```python
from build123d import *

# Parameters (mm, degrees)
SKETCH1_W           = 23.056445047489827
SKETCH1_H           = 95.25
SKETCH1_R           = 1.2700000000000005
SKETCH1_R_2         = 1.269999999999998
BOSS_EXTRUDE1_DEPTH = 6.35
SKETCH2_W           = 23.056445047489827
SKETCH2_H           = 48.26
BOSS_EXTRUDE2_DEPTH = 12.7
CUT_EXTRUDE2_DEPTH  = 55.41534970233967
SKETCH6_R           = 3.4289999999999994
CUT_EXTRUDE3_DEPTH  = 53.57321599024526
FILLET2_R           = 1.27
BOSS_EXTRUDE3_DEPTH = 6.35
SKETCH9_R           = 1.9049999999999996
SKETCH9_R_2         = 1.905
CUT_EXTRUDE4_DEPTH  = 53.43149307056342
FILLET4_R           = 2.54
BOSS_EXTRUDE7_DEPTH = 6.35
FILLET5_R           = 2.54
FILLET6_R           = 2.54
SKETCH13_R          = 2.0319999999999987
SKETCH13_R_2        = 2.032000000000001
CUT_EXTRUDE5_DEPTH  = 6.35
FILLET7_R           = 2.54


with BuildPart() as part:
    # Sketch1 → Boss-Extrude1 (new body)
    # profile 1 of 4: a face of its own
    with BuildSketch(Plane.XY):
        Rectangle(SKETCH1_W, SKETCH1_H)
        Polygon((7.9121000000000015, 16.687800000000006), (7.9121000000000015, 44.449999999999996), (-7.912099999999998, 44.45), (-7.912099999999998, 16.687800000000006), align=None, mode=Mode.SUBTRACT)
    # profile 2 of 4: a face of its own
    with BuildSketch(Plane.XY):
        Polygon((-7.912099999999998, 16.687800000000006), (7.9121000000000015, 16.687800000000006), (7.9121000000000015, 44.449999999999996), (-7.912099999999998, 44.45), align=None)
        with Locations((5.372100000000001, 19.227800000000006)):
            Circle(SKETCH1_R, mode=Mode.SUBTRACT)
        with Locations((-5.372099999999998, 41.910000000000004)):
            Circle(SKETCH1_R_2, mode=Mode.SUBTRACT)
    # profile 3 of 4: a face of its own
    with BuildSketch(Plane.XY):
        with Locations((-5.372099999999998, 41.910000000000004)):
            Circle(SKETCH1_R_2)
    # profile 4 of 4: a face of its own
    with BuildSketch(Plane.XY):
        with Locations((5.372100000000001, 19.227800000000006)):
            Circle(SKETCH1_R)
    extrude(amount=BOSS_EXTRUDE1_DEPTH)

    # Sketch2 → Boss-Extrude2 (add)
    with BuildSketch(Plane(origin=(0, 0, 0), x_dir=(-1, 0, 0), z_dir=(0, 0, -1))):
        with Locations((0, -23.495)):
            Rectangle(SKETCH2_W, SKETCH2_H)
    extrude(amount=BOSS_EXTRUDE2_DEPTH)

    # Sketch5 → Cut-Extrude2 (cut, through all)
    with BuildSketch(Plane(origin=(11.528222523744914, 0, 0), x_dir=(0, 0, -1), z_dir=(1, 0, 0))):
        Polygon((-0.6350000000000019, -12.065000000000001), (9.524999999999997, -12.065000000000001), (9.524999999999999, -8.255000000000003), (-0.6350000000000019, -8.255000000000003), align=None)
    extrude(amount=-CUT_EXTRUDE2_DEPTH, mode=Mode.SUBTRACT)

    # Sketch6 → Cut-Extrude3 (cut, through all)
    with BuildSketch(Plane(origin=(0, 0, -12.7), x_dir=(-1, 0, 0), z_dir=(0, 0, -1))):
        with Locations((0, -28.575)):
            Circle(SKETCH6_R)
    extrude(amount=-CUT_EXTRUDE3_DEPTH, mode=Mode.SUBTRACT)

    # Fillet2
    fillet2_edges = [part.edges().sort_by_distance(p)[0] for p in [
        (-11.528222523744914, -10.160000000000004, -9.524999999999999),
        (0, -8.255000000000003, -9.524999999999999),
        (-11.528222523744914, -12.065, -4.444999999999998),
        (0, -12.065000000000001, -9.524999999999997),
        (-11.528222523744914, -10.16, 0.6350000000000019),
        (0, -12.065000000000001, 0.6350000000000019),
        (-11.528222523744914, -8.255000000000003, -4.4449999999999985),
        (0, -8.255000000000003, 0.6350000000000019),
        (11.528222523744914, -10.160000000000002, -9.524999999999999),
        (11.528222523744914, -8.255000000000003, -4.4449999999999985),
        (11.528222523744914, -10.160000000000002, 0.6350000000000019),
        (11.528222523744914, -12.065000000000001, -4.444999999999998),
    ]]
    fillet(fillet2_edges, radius=FILLET2_R)

    # Sketch8 → Boss-Extrude3 (add)
    with BuildSketch(Plane.ZY.offset(11.528222523744914)):
        Polygon((6.35, 47.625), (-1.21e-15, 47.625), (0, 6.98625472546675), (6.350000000000005, 6.986254725466751), align=None)
    extrude(amount=BOSS_EXTRUDE3_DEPTH)

    # Sketch9 → Cut-Extrude4 (cut, through all)
    with BuildSketch(Plane.XY):
        with Locations((-4.594022523744915, 12.877800000000006)):
            Circle(SKETCH9_R)
        with Locations((-15.338222523744914, 35.56)):
            Circle(SKETCH9_R_2)
    extrude(amount=CUT_EXTRUDE4_DEPTH, mode=Mode.SUBTRACT)

    # Fillet4
    fillet4_edges = [part.edges().sort_by_distance(p)[0] for p in [
        (11.528222523744914, 47.625, 3.175),
        (-11.528222523744914, 6.98625472546675, 3.1750000000000025),
        (-17.878222523744913, 47.625, 3.1749999999999994),
        (-17.878222523744913, 6.98625472546675, 3.1750000000000025),
    ]]
    fillet(fillet4_edges, radius=FILLET4_R)

    # Sketch12 → Boss-Extrude7 (add)
    with BuildSketch(Plane(origin=(11.528222523744914, 0, 0), x_dir=(0, 0, -1), z_dir=(1, 0, 0))):
        Polygon((-6.35, 0.6349999999999898), (18.613653389650153, 0.6349999999999898), (18.613653389650153, 9.627193152709879), (-17.78195834691587, 9.627193152709879), (-17.78195834691587, 0.6349999999999898), align=None)
    extrude(amount=-BOSS_EXTRUDE7_DEPTH)

    # Fillet5
    fillet5_edges = [part.edges().sort_by_distance(p)[0] for p in [
        (8.353222523744913, 0.6349999999999967, -12.7),
        (8.353222523744915, 9.627193152709879, 6.3500000000000005),
        (8.353222523744915, 9.627193152709879, 0),
        (5.178222523744914, 5.131096576354938, 0),
        (8.353222523744915, 0.6349999999999898, 6.35),
    ]]
    fillet(fillet5_edges, radius=FILLET5_R)

    # Fillet6
    fillet6_edges = [part.edges().sort_by_distance(p)[0] for p in [
        (5.178222523744914, -0.6350000000000069, -12.7),
    ]]
    fillet(fillet6_edges, radius=FILLET6_R)

    # Sketch13 → Cut-Extrude5 (cut)
    with BuildSketch(Plane(origin=(11.528222523744914, 0, 0), x_dir=(0, 0, -1), z_dir=(1, 0, 0))):
        with Locations((-12.70195834691587, 5.050717249087455)):
            Circle(SKETCH13_R)
        with Locations((12.698041653084129, 5.050717249087455)):
            Circle(SKETCH13_R_2)
    extrude(amount=-CUT_EXTRUDE5_DEPTH, mode=Mode.SUBTRACT)

    # Fillet7
    fillet7_edges = [part.edges().sort_by_distance(p)[0] for p in [
        (8.353222523744915, 0.6349999999999898, -18.613653389650153),
        (8.353222523744915, 0.6349999999999898, 17.78195834691587),
        (8.353222523744915, 9.627193152709879, 17.78195834691587),
        (8.353222523744915, 9.627193152709879, -18.613653389650153),
    ]]
    fillet(fillet7_edges, radius=FILLET7_R)


solid = part.part
```
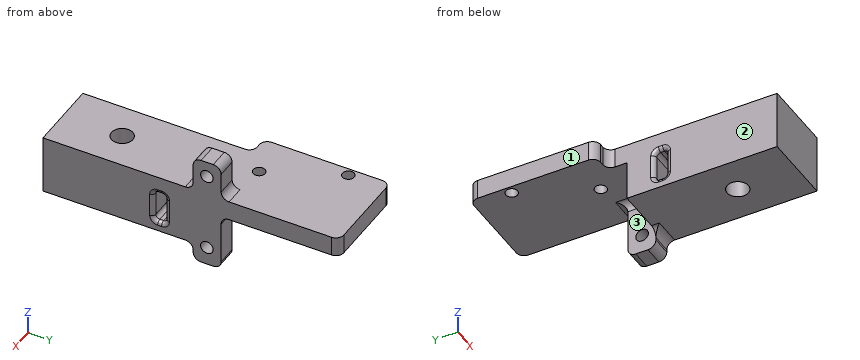
Geometry: final body of the model. Coordinates: model frame, mm. Face numbers are marked on the shaded views. A direction names the side the tool comes from. Coordinates: 2 decimals unless noted, no trailing zeros. Write each loop counter-clockwise with the first axis right and the second up, starting at its lowest first coordinate (ties: lowest second). Pieces come first, ordered by that corner, then holes. Notation, with made-up numbers: M 20,5.5 L 65,5.5 A20 cw 65,29.5 Z; hole C -22.75,45 d9. An arc over 180 degrees is marked long. Answer as CSV lines item,"result". Start each with the question number.
Q1. Pin query (flat end, axial travel): P1, Ø10, axis at x = 6.5, y = 33, coming from the +Z side; P2, Ø1.9, axis at x = 9, z = -10, coming from the +Y side; P3, Ø0.6, axis at x = -14.5, z = 4.5, coming from the -Y side. Return the tip coordinate at first contact, or that it passes through.
Q2. Cut plane A-A on x = 0. Return the cut outline in (y, z) (3 decimals), then the cut area to 3 significant figures.
Q3. Line query: line 1 (Y direction, x = 0, z = -2.25) (3 decimals); line 2 (Z direction, x = -9.75, y = 11); line 3 (Z direction, x = -3.5, y = -40). Output: solid intervals per line, ascending. Write a range as from..to.
Q4. Reachability of the marked faces 1, 2 and 3 from +Z, -Z, +X, -X, +Y, -Y: full face, straight path, thin tool, end or side. Return the list, or none.
Q5. Cut plane C-C on z = 3.5. Return the cut outline in (x, y) (3 decimals).
Q6. Cut plane B-B on y = 35.56. Return the cut outline in (x, z), then the cut area to 3 significant figures.
Findings below:
1,P1,"stops at z = 6.35"
1,P2,"stops at y = 9.63"
1,P3,"stops at y = 6.99"
2,outline,"M -47.625,-12.7 L -32.004,-12.7 L -32.004,6.35 L -47.625,6.35 Z; M -25.146,-12.7 L 0.635,-12.7 L 0.635,0 L 47.625,0 L 47.625,6.35 L -25.146,6.35 Z; hole M -12.065,-8.255 A1.27 ccw -10.795,-9.525 L -9.525,-9.525 A1.27 ccw -8.255,-8.255 L -8.255,-0.635 A1.27 ccw -9.525,0.635 L -10.795,0.635 A1.27 ccw -12.065,-0.635 Z"
2,area,"1,050 mm2"
3,line 1,"y = -47.625..-32.004, -25.146..-12.065, -8.255..0.635"
3,line 2,"z = 0..6.35"
3,line 3,"z = -12.7..6.35"
4,face 1,"+Z, -Z, -X, +Y, -Y"
4,face 2,"+Z, -Z, -X, -Y"
4,face 3,"-Z, -X, +Y"
5,outline,"M -17.878,9.526 A2.54 ccw -15.338,6.986 L -14.068,6.986 A2.54 cw -11.528,4.446 L -11.528,-47.625 L 11.528,-47.625 L 11.528,45.085 A2.54 ccw 8.988,47.625 L -15.338,47.625 A2.54 ccw -17.878,45.085 Z; hole C -15.338,35.56 d3.81; hole C -4.594,12.878 d3.81; hole C 0,-28.575 d6.858"
6,outline,"M -17.88,0 L -17.24,0 L -17.24,6.35 L -17.88,6.35 Z; M -13.43,0 L 11.53,0 L 11.53,6.35 L -13.43,6.35 Z"
6,area,"163 mm2"
